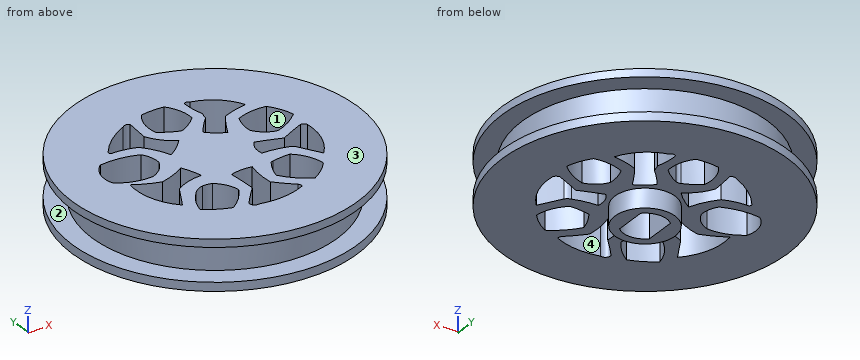
Autodesk Inventor part; units mm, degrees
ref_plane "YZ Plane" through (0, 0, 0) normal (1, 0, 0) x (0, 1, 0)
ref_plane "XZ Plane" through (0, 0, 0) normal (0, 1, 0) x (-1, 0, 0)
ref_plane "XY Plane" through (0, 0, 0) normal (0, 0, 1) x (1, 0, 0)
sketch "Sketch1" plane through (0, 0, 0) normal (0, 0, 1) x (1, 0, 0)
  circle A0 centre (0, 0) radius 4.826
  dimension "d0" = 9.652
extrude "Extrusion1" add sketch "Sketch1" along normal blind 3.048
sketch "Sketch2" plane through (0, 0, 3.048) normal (0, 0, 1) x (1, 0, 0)
  circle A0 centre (0, 0) radius 22.86
  dimension "d3" = 45.72
extrude "Extrusion2" add sketch "Sketch2" along normal blind 1.397
sketch "Sketch4" plane through (0, 0, 4.445) normal (0, 0, 1) x (1, 0, 0)
  circle A0 centre (0, 0) radius 19.685
  dimension "d6" = 39.37
extrude "Extrusion3" add sketch "Sketch4" along normal blind 5.334
sketch "Sketch6" plane through (0, 0, 9.779) normal (0, 0, 1) x (1, 0, 0)
  circle A0 centre (0, 0) radius 4.826
  circle A1 centre (0, 0) radius 22.86
extrude "Extrusion4" add sketch "Sketch6" along normal blind 1.27 contours A0 | A1
sketch "Sketch9" plane through (0, 0, 0) normal (0, 0, -1) x (-1, 0, 0)
  line L0 (2.3876, -2.514) -> (2.3876, 2.514)
  line L1 (-2.3876, 2.514) -> (-2.3876, -2.514)
  line L2 (-1.2735, -3.2247) -> (1.2735, 3.2247) construction
  line L3 (1.2735, -3.2247) -> (-1.2735, 3.2247) construction
  arc A0 (-2.3876, -2.514) -> (2.3876, -2.514) centre (0, 0) ccw
  arc A1 (2.3876, 2.514) -> (-2.3876, 2.514) centre (0, 0) ccw
extrude "Extrusion6" cut sketch "Sketch9" against normal blind 5.5118
sketch "Sketch10" plane through (0, 0, 3.048) normal (0, 0, -1) x (-1, 0, 0)
  arc A0 (6.0888, 12.8089) -> (4.9517, 12.8553) centre (5.4971, 12.2636) ccw
  arc A1 (11.5392, 8.311) -> (6.0888, 12.8089) centre (0.4834, 0.4651) ccw
  arc A2 (11.0546, 7.7734) -> (11.5392, 8.311) centre (11.2368, 8.0964) ccw
  arc A3 (11.0546, 7.7734) -> (7.4347, 7.1004) centre (11.1442, -2.7813) ccw
  circle A4 centre (0, 0) radius 22.86
  arc A5 (5.2433, 9.0758) -> (4.9517, 12.8553) centre (-169.1009, -2.4734) ccw
  arc A6 (2.0036, 5.6242) -> (5.2433, 9.0758) centre (-1.766, 12.4088) ccw
  arc A7 (2.0036, 5.6242) -> (4.9517, 3.0409) centre (11.897, 13.941) ccw
  arc A8 (7.4347, 7.1004) -> (4.9517, 3.0409) centre (16.2062, -1.0536) ccw
  arc A9 (11.2368, -8.9724) -> (14.0004, -0.5744) centre (4.7112, -2.1713) ccw
  arc A10 (9.1497, -5.1175) -> (11.2368, -8.9724) centre (208.9836, 100.5866) ccw
  arc A11 (9.1497, -5.1175) -> (4.7112, -3.7562) centre (4.4946, -12.3784) ccw
  arc A12 (5.8832, -0.5744) -> (4.7112, -3.7562) centre (18.9185, -7.1827) ccw
  arc A13 (5.8832, -0.5744) -> (9.9506, -2.3296) centre (12.8849, 10.061) ccw
  arc A14 (9.9506, -2.3296) -> (14.0004, -0.5744) centre (5.7085, 13.0084) ccw
  arc A15 (9.9506, -11.266) -> (7.84, -7.1827) centre (1.8046, -12.8894) ccw
  arc A16 (7.84, -7.1827) -> (6.2065, -6.2202) centre (5.7633, -8.8398) ccw
  arc A17 (6.2065, -6.2202) -> (4.6733, -6.4168) centre (5.7633, -8.8398) ccw
  arc A18 (4.6733, -6.4168) -> (2.7073, -9.6817) centre (7.7197, -10.4756) ccw
  arc A19 (2.7073, -9.6817) -> (5.9896, -13.3063) centre (11.6592, -4.8738) ccw
  arc A20 (5.9896, -13.3063) -> (9.9506, -11.266) centre (2.5555, -1.7743) ccw
  arc A21 (1.2488, -5.7954) -> (-2.1893, -5.6065) centre (-0.8542, -12.6863) ccw
  arc A22 (1.2488, -5.7954) -> (0.9545, -10.3074) centre (53.2412, -11.4518) ccw
  arc A23 (3.6527, -13.5111) -> (0.9545, -10.3074) centre (-39.0545, -46.7416) ccw
  arc A24 (2.5555, -14.4106) -> (3.6527, -13.5111) centre (2.8151, -13.6083) ccw
  arc A25 (-4.8162, -13.6083) -> (2.5555, -14.4106) centre (0.014, -3.4952) ccw
  arc A26 (-4.6201, -12.8894) -> (-4.8162, -13.6083) centre (-4.1772, -13.3965) ccw
  arc A27 (-4.6201, -12.8894) -> (-1.9227, -10.3074) centre (-21.7976, 7.7557) ccw
  arc A28 (-1.9227, -10.3074) -> (-2.1893, -5.6065) centre (-14.7824, -8.6787) ccw
  arc A29 (-7.4482, -12.7759) -> (-3.5507, -9.27) centre (-12.4495, -3.2965) ccw
  arc A30 (-3.5507, -9.27) -> (-4.8162, -6.2202) centre (-13.041, -11.4205) ccw
  arc A31 (-4.8162, -6.2202) -> (-5.2818, -5.9098) centre (-5.2043, -6.2979) ccw
  arc A32 (-5.2818, -5.9098) -> (-8.2329, -5.6065) centre (-7.9223, -17.09) ccw
  arc A33 (-8.2329, -5.6065) -> (-10.6197, -10.0458) centre (-4.1164, -10.6809) ccw
  arc A34 (-10.6197, -10.0458) -> (-7.4482, -12.7759) centre (-2.1705, -3.4378) ccw
  arc A35 (2.3346, 14.0815) -> (-1.3832, 14.2076) centre (0.0752, 2.3347) ccw
  arc A36 (3.3497, 9.1954) -> (2.3346, 14.0815) centre (-2.4317, 10.5428) ccw
  arc A37 (0.5801, 7.6979) -> (3.3497, 9.1954) centre (-3.4245, 18.4144) ccw
  arc A38 (-2.849, 9.7313) -> (-0.2799, 7.7734) centre (3.746, 15.7205) ccw
  arc A39 (-1.3832, 14.2076) -> (-2.849, 9.7313) centre (3.0799, 10.268) ccw
  arc A40 (-4.6201, 3.8276) -> (-1.9227, 5.7208) centre (-7.3541, 10.5911) ccw
  arc A41 (-4.6201, 3.8276) -> (-6.7475, 7.596) centre (-37.5112, -12.2565) ccw
  arc A42 (-1.9227, 5.7208) -> (-4.3382, 8.6929) centre (-18.3879, -5.1934) ccw
  arc A43 (-4.3382, 8.6929) -> (-4.6201, 9.8732) centre (-8.7751, 8.2571) ccw
  arc A44 (-4.6201, 9.8732) -> (-4.1164, 13.3822) centre (-15.2899, 13.1953) ccw
  arc A45 (-4.1164, 13.3822) -> (-4.9848, 13.3822) centre (-4.5506, 13.1456) ccw
  arc A46 (-4.9848, 13.3822) -> (-10.7538, 8.6929) centre (-3.2343, 5.3353) ccw
  arc A47 (-6.7475, 7.596) -> (-10.7538, 8.6929) centre (-12.3706, -5.0773) ccw
  arc A48 (-7.9223, 6.0993) -> (-12.7557, 6.7633) centre (-11.4073, -1.3439) ccw
  arc A49 (-7.3541, 2.6988) -> (-7.9223, 6.0993) centre (-14.7929, 3.2035) ccw
  arc A50 (-10.4577, 0.4986) -> (-7.3541, 2.6988) centre (-11.2012, 4.8363) ccw
  arc A51 (-14.5898, 3.0409) -> (-10.4577, 0.4986) centre (-7.2589, 10.3268) ccw
  arc A52 (-12.7557, 6.7633) -> (-14.5898, 3.0409) centre (-5.9799, 1.1117) ccw
  arc A53 (-5.2818, -3.2965) -> (-6.0542, -0.2883) centre (-8.5618, -2.5354) ccw
  arc A54 (-6.0542, -0.2883) -> (-10.0183, -1.5931) centre (9.876, -55.3624) ccw
  arc A55 (-5.2818, -3.2965) -> (-9.1684, -3.8787) centre (-5.1947, -17.1417) ccw
  arc A56 (-9.1684, -3.8787) -> (-10.0183, -4.397) centre (-8.8628, -5.3359) ccw
  arc A57 (-10.0183, -1.5931) -> (-13.8141, 0.2266) centre (-38.6644, -56.4801) ccw
  arc A58 (-13.8141, 0.2266) -> (-14.5898, -0.2883) centre (-13.7445, -0.72) ccw
  arc A59 (-14.5898, -0.2883) -> (-12.122, -7.8577) centre (-4.7204, -1.2577) ccw
  arc A60 (-12.122, -7.8577) -> (-10.0183, -4.397) centre (-273.7033, 153.5242) ccw
  arc A61 (-0.2799, 7.7734) -> (0.5801, 7.6979) centre (0.2215, 8.5495) ccw
  arc A62 (8.3209, 5.3046) -> (7.4347, 2.3347) centre (11.6708, 2.6878) ccw
  arc A63 (7.4347, 2.3347) -> (10.2097, -0.443) centre (11.8697, 3.9904) ccw
  arc A64 (14.3339, 6.0011) -> (8.3209, 5.3046) centre (12.587, -5.2209) ccw
  arc A65 (15.6088, 1.087) -> (14.3339, 6.0011) centre (11.6708, 2.6878) ccw
  arc A66 (10.2097, -0.443) -> (15.6088, 1.087) centre (10.9403, 7.27) ccw
extrude "Extrusion7" cut sketch "Sketch10" against normal through all contours A1 A2 A3 A8 A7 A6 A5 A0 | A10 A11 A12 A13 A14 A9 | A20 A19 A18 A17 A16 A15 | A22 A23 A24 A25 A26 A27 A28 A21 | A34 A33 A32 A31 A30 A29 | A36 A37 A61 A38 A39 A35 | A41 A47 A46 A45 A44 A43 A42 A40 | A49 A50 A51 A52 A48 | A55 A56 A60 A59 A58 A57 A54 A53 | A64 A65 A66 A63 A62
properties part number "Desgin on wheel"
Here's how the part is built. I have some questions about the finished solid (model axes, mm). Face numbers are marked on the shaded views. A direction names the side the tool comes from. Give positions to 0.01 mm unless a question says otherwise; leave off trailing zeros. Write each loop counter-clockwise with the first axis right and the second up, starting at its lowest first coordinate (ties: lowest second). Pieces come first, ordered by that corner, then holes. Notation, with made-up numbers: M 6,-36.5 L 37,-36.5 A12 cw 37,-17.5 Z; hole C -13,-38 d1. An arc over 180 degrees is marked long. Put each result on its own line as item: value. Start each with the question number.
Item 1: Thinking about a two-plate mould opening in Y: for the marked faces 1 and 2, which applies, +Y half, -Y half, draft (parallel to the pull), parting line (faces both ways), or undercut?
Item 2: If we section it at A-A, the plane y = 10.5: Write out the boundary of the cut face in (x, z) (3 decimals).
Item 3: If we section it at C-C, the plane z = 6.5: Count the separate pieces of the cut face and the enclosed holes in it, then the cut area to 3 significant figures.
Item 4: Will these pins go through, and if not, where does the flat tip stop? pin 1 (1.5 mm diameter, centred on y = 16.5, z = 3.5, fed in from +X); pin 2 (1.5 mm diameter, centred on x = 11.5, z = 10, fed in from -Y); pin 3 (2 mm diameter, centred on x = -9, z = 3, fed in from +Y).
Item 5: On a 3-axis mill with a long thin cutter (end or side, diameter ignored), from which of +Z, -Z, +X, -X, +Y, -Y can I reach the whole of each face in a straight line? I mean the marked faces 3 and 4. Say none if no direction works.
Item 6: If we section it at B-B, the plane x = -19: Write out the boundary of the cut face in (y, z) (3 decimals), then the cut area to 3 significant figures.
Item 7: I need wall thicknesses on L1, parallel to X at y = 4.5, z = 10.75; L2, parallel to Z at x = -6, y = -19 (3 decimals); L3, parallel to X at y = -11, z = 3.25. Which ranges of each line are inside material? Lowest first, please. Write a range as from..to.
Values:
1. face 1: undercut
1. face 2: draft
2. outline: M -20.306,3.048 L -9.599,3.048 L -9.599,11.049 L -20.306,11.049 L -20.306,9.779 L -16.651,9.779 L -16.651,4.445 L -20.306,4.445 Z; M -5.143,3.048 L -3.504,3.048 L -3.504,11.049 L -5.143,11.049 Z; M 2.869,3.048 L 4.445,3.048 L 4.445,11.049 L 2.869,11.049 Z; M 9.649,3.048 L 20.306,3.048 L 20.306,4.445 L 16.651,4.445 L 16.651,9.779 L 20.306,9.779 L 20.306,11.049 L 9.649,11.049 Z
3. separate pieces: 1
3. enclosed holes: 10
3. area: 843 mm²
4. pin 1: x = 16.57
4. pin 2: y = -20.17
4. pin 3: y = 21.41
5. face 3: +Z, +X, -X, +Y, -Y
5. face 4: +Z, -Z
6. outline: M -12.711,3.048 L 12.711,3.048 L 12.711,4.445 L 5.148,4.445 L 5.148,9.779 L 12.711,9.779 L 12.711,11.049 L -12.711,11.049 L -12.711,9.779 L -5.148,9.779 L -5.148,4.445 L -12.711,4.445 Z
6. area: 123 mm²
7. L1: -22.41..-15.52, -7.83..-5.6, -3.07..3.34, 4.96..7.45, 14.13..22.41
7. L2: 3.048..4.445, 9.779..11.049
7. L3: -20.04..-9.89, -3.55..-1.57, 2.57..5, 9.78..20.04
